```python
from build123d import *

# Parameters (mm, degrees)
F0_W     = 300
F0_H     = 430
F1_DEPTH = 1
F2_W     = 300
F2_H     = 1
F3_DEPTH = 100
F4_W     = 1
F4_H     = 430
F5_DEPTH = 100
F6_W     = 1
F6_H     = 430
F7_DEPTH = 100


with BuildPart() as f1:
    # F0 (on Top) → F1 (new body)
    with BuildSketch(Plane.XY):
        Rectangle(F0_W, F0_H)
    extrude(amount=-F1_DEPTH)

    # F2 (on Top) → F3 (join)
    with BuildSketch(Plane.XY):
        with Locations((0.038886, 214.259856)):
            Rectangle(F2_W, F2_H)
    extrude(amount=F3_DEPTH)

    # F4 (on Top) → F5 (join)
    with BuildSketch(Plane.XY):
        with Locations((147.787129, -0.097331)):
            Rectangle(F4_W, F4_H)
    extrude(amount=F5_DEPTH)

    # F6 (on Top) → F7 (join)
    with BuildSketch(Plane.XY):
        with Locations((-150.013192, 0.495426)):
            Rectangle(F6_W, F6_H)
    extrude(amount=F7_DEPTH)


solid = f1.part
```
For this review, take the finished solid that the model builds, in its own axes (mm). A direction names the side the tool comes from. Coordinates: 2 decimals unless noted, no trailing zeros. Write each loop counter-clockwise with the first axis right and the second up, starting at its lowest first coordinate (ties: lowest second). Pieces come first, ordered by that corner, then holes.
(1) Add section A-A on y = 151. Give the boundary of the cut face in (x, z).
(2) The part is to be moulded in two halves that separate along X. For faces 1 (the face through (147.287, -4, 49)), 2 (the face through (-2, 3, -1)), 3 (the face through (-150.513, -3, 49)), say which applies: +X half, -X half, draft (parallel to the pull), parting line (faces both ways), or undercut.
(3) Tool access review of faces 4 (the face through (-149.513, -3, 49)), 5 (the face through (148.287, -4, 49)): name each direction out of +Z, -Z, +X, -X, +Y, -Y from which nothing blocks a thin tool from reaching the whole face with its end or side.
(4) Add section C-C on x = -92.5. Give the boundary of the cut face in (y, z).
(5) Add section B-B on z = 62. Give the boundary of the cut face in (x, y), then the cut area to 3 significant figures.
(6) Wall thickness on probe 1 along X at (y, z) = (191.5, 6); probe 2 along Z at (x, y) = (80, -54.5); probe 3 along Y at (x, z) = (11.5, 31.5): over which ranges is each line inside the solid? List them lowest first.
(7) For pin 1 Ø3 at (x, z) = (-69, 86.5) entering from +Y; pin 2 Ø0.5 at (x, z) = (8, -0.5) entering from +Y; pin 3 Ø1.5 at (x, y) = (-25, -163.5) entering from +Z, all flat-tipped, find the tip position at first contact; note any pin that passes through.
Answer sheet:
1. outline: (-150.51, 0) - (-150, 0) - (-150, -1) - (150, -1) - (150, 0) - (148.29, 0) - (148.29, 100) - (147.29, 100) - (147.29, 0) - (-149.51, 0) - (-149.51, 100) - (-150.51, 100) - close
2. face 1: undercut
2. face 2: draft
2. face 3: -X half
3. face 4: +Z, -Y
3. face 5: +Z, +X, -Y
4. outline: (-215, -1) - (215, -1) - (215, 0) - (214.76, 0) - (214.76, 100) - (213.76, 100) - (213.76, 0) - (-215, 0) - close
5. outline: (-150.51, -214.5) - (-149.51, -214.5) - (-149.51, 213.76) - (147.29, 213.76) - (147.29, -215.1) - (148.29, -215.1) - (148.29, 213.76) - (150.04, 213.76) - (150.04, 214.76) - (148.29, 214.76) - (148.29, 214.9) - (147.29, 214.9) - (147.29, 214.76) - (-149.51, 214.76) - (-149.51, 215.5) - (-150.51, 215.5) - close
5. area: 1,160 mm2
6. probe 1: x = -150.51 to -149.51, 147.29 to 148.29
6. probe 2: z = -1 to 0
6. probe 3: y = 213.76 to 214.76
7. pin 1: stops at y = 214.76
7. pin 2: stops at y = 215
7. pin 3: stops at z = 0
